Study the drawing (mm; zero at the part's minimum x, y, z) and answer. Give positions to 0.01 mm unless a question says otherwise; leave off trailing zeros. Write each loop counter-clockwise with the first axis right and the second up, starting at its lowest first coordinate (ties: lowest second). Pieces come first, ordered by that corner, then holes.
1) Find section A-A (x = 30). Determine the outline of the cut face in (y, z).
2) Find section D-D (z = 6). Determine the outline of the cut face in (x, y).
3) Given pin 1 Ø5 at (x, z) = (30, 30) entering from -Y; pin 2 Ø1 at (x, y) = (33, 3) entering from +Z; pin 3 Ø1.6 at (y, z) = (1, 29) entering from -X; pin 4 Ø1 at (x, y) = (31.5, 1) entering from +Z, each flat-ended and moving along its own axis, determine where each tip first touches the part or whether it passes through.
4) Find section C-C (y = 0.9). Determine the outline of the cut face in (x, z), plus the area to 3 significant figures.
5) Straight lines are drawn through the part: probe 1 along X at (y, z) = (1.25, 30); probe 2 along X at (y, z) = (3, 30). For each, find the intervals that lie inside material, in ascending order.
6) Find section B-B (z = 30). Determine the outline of the cut face in (x, y), plus the area to 3 significant figures.
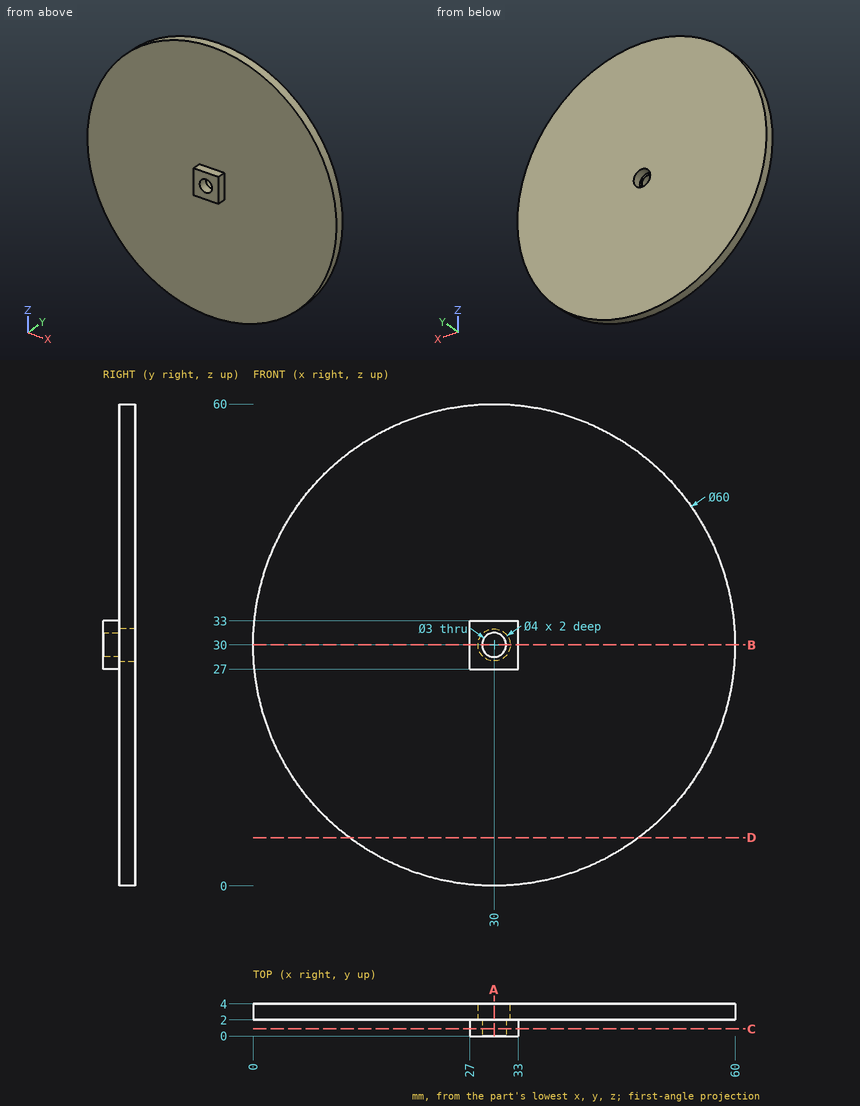
Results:
1. outline: (0, 27) - (2, 27) - (2, 0) - (4, 0) - (4, 28) - (2, 28) - (2, 28.5) - (0, 28.5) - close; (0, 31.5) - (2, 31.5) - (2, 32) - (4, 32) - (4, 60) - (2, 60) - (2, 33) - (0, 33) - close
2. outline: (12, 2) - (48, 2) - (48, 4) - (12, 4) - close
3. pin 1: stops at y = 0
3. pin 2: stops at z = 59.9
3. pin 3: stops at x = 27
3. pin 4: stops at z = 33
4. outline: (27, 27) - (33, 27) - (33, 33) - (27, 33) - close; hole circle Ø3 at (30, 30)
4. area: 28.9 mm2
5. probe 1: x = 27 to 28.5, 31.5 to 33
5. probe 2: x = 0 to 28, 32 to 60
6. outline: (0, 2) - (27, 2) - (27, 0) - (28.5, 0) - (28.5, 2) - (28, 2) - (28, 4) - (0, 4) - close; (31.5, 0) - (33, 0) - (33, 2) - (60, 2) - (60, 4) - (32, 4) - (32, 2) - (31.5, 2) - close
6. area: 118 mm2
